Build history of the part. All positions in model axes, mm. A direction names the side the tool comes from. Give positions to 0.01 mm unless a question says otherwise; leave off trailing zeros. Write each loop counter-clockwise with the first axis right and the second up, starting at its lowest first coordinate (ties: lowest second). Pieces come first, ordered by that corner, then holes. Notation, with made-up numbers: M 64.5,52.5 L 90.5,52.5 A21 cw 90.5,57.5 Z; hole C -39,-11.5 d6. An arc over 180 degrees is marked long. Return JSON: item names as keys, results as strings. Group by question number.
Q1. Wall check: probe 1 along X at (y, z) = (36, 8) (3 decimals); probe 2 along Y at (x, z) = (11.1, 0). Give the ranges that are in metal, low to high.
Q2. Band-saw the part on D-D, the plane y = 54. Give the cut face in (x, z) (3 decimals).
Q3. Band-saw the part on C-C, the plane z = 0. Give the cut face in (x, y) (3 decimals), then the cut area to 3 significant figures.
Q4. Band-saw the part on B-B, the plane y = 12.7. Give the cut face in (x, z) (3 decimals), then the cut area to 3 significant figures.
Q5. Pull direction X, two halves, no side cores. Call faces 3 (the flat face through (-12.7, 138, 0)), 4 (the flat face through (0, 138, 9.525)), 5 (the cylindrical face through (-11.09, 15.924, 0.423)): +X half, -X half, draft (parallel to the pull), parting line (faces both ways), or undercut.
Q6. Tool access for faces 1 (the flat face through (12.7, 138, 0)), 2 (the flat face through (0, 138, -9.525)): list every direction of +Z, -Z, +X, -X, +Y, -Y with a clear straight run to the whole face (end or side of a thin tool).
Q7. Flat gauge pins, fed straight in: pin 1 Ø10.5 at (y, z) = (12.7, 0) entering from +X; pin 2 Ø3 at (x, z) = (-6.5, -2.5) entering from -Y (3 decimals). Where does each tip first touch, or does it go through?
Q8. Band-saw the part on A-A, the plane x = -1.75. Give the cut face in (y, z) (3 decimals), then the cut area to 3 significant figures.
Autodesk Inventor part; units mm, degrees
ref_plane "YZ Plane" through (0, 0, 0) normal (1, 0, 0) x (0, 1, 0)
ref_plane "XZ Plane" through (0, 0, 0) normal (0, 1, 0) x (-1, 0, 0)
ref_plane "XY Plane" through (0, 0, 0) normal (0, 0, 1) x (1, 0, 0)
sketch "Sketch1" plane through (0, 0, 0) normal (0, 1, 0) x (-1, 0, 0)
  line L0 (-12.7, -12.7) -> (12.7, -12.7)
  line L1 (12.7, -12.7) -> (12.7, 12.7)
  line L2 (12.7, 12.7) -> (-12.7, 12.7)
  line L3 (-12.7, 12.7) -> (-12.7, -12.7)
  line L4 (-12.7, -12.7) -> (12.7, 12.7) construction
  line L5 (12.7, -12.7) -> (-12.7, 12.7) construction
  line L6 (9.525, 9.525) -> (9.525, -9.525)
  line L7 (9.525, -9.525) -> (-9.525, -9.525)
  line L8 (-9.525, -9.525) -> (-9.525, 9.525)
  line L9 (-9.525, 9.525) -> (9.525, 9.525)
  point P0 (0, 0)
  dimension "d0" = 25.4
  dimension "d1" = 25.4
  dimension "d2" = 3.175
extrude "Extrusion1" add sketch "Sketch1" along normal blind 279.4
sketch "Sketch2" plane through (12.7, 0, 12.7) normal (1, 0, 0) x (0, 0, -1)
  circle A0 centre (12.7, 12.7) radius 3.2512
  line L0 (0, 0) -> (25.4, 0)
  point P0 (12.7, 0)
  point P1 (12.7, 0)
  point P2 (12.7, 0)
  dimension "d5" = 6.5024
  dimension "d6" = 12.7
extrude "Extrusion2" cut sketch "Sketch2" against normal blind 25.4
properties part number "STRU_010_BilletPole_11in_Unique" material "Aluminum 6061"
From the geometry:
{
 "1": {"probe 1": "x = -12.7 to -9.525, 9.525 to 12.7", "probe 2": "y = 0 to 9.45, 15.95 to 279.4"},
 "2": {"outline": "M -12.7,-12.7 L 12.7,-12.7 L 12.7,12.7 L -12.7,12.7 Z; hole M -9.525,-9.525 L 9.525,-9.525 L 9.525,9.525 L -9.525,9.525 Z"},
 "3": {"outline": "M -12.7,0 L -9.525,0 L -9.525,9.449 L -12.7,9.449 Z; M -12.7,15.951 L -9.525,15.951 L -9.525,279.4 L -12.7,279.4 Z; M 9.525,0 L 12.7,0 L 12.7,9.449 L 9.525,9.449 Z; M 9.525,15.951 L 12.7,15.951 L 12.7,279.4 L 9.525,279.4 Z", "area": "1,730 mm^2"},
 "4": {"outline": "M -12.7,-12.7 L 12.7,-12.7 L 12.7,-3.251 L 9.525,-3.251 L 9.525,-9.525 L -9.525,-9.525 L -9.525,-3.251 L -12.7,-3.251 Z; M -12.7,3.251 L -9.525,3.251 L -9.525,9.525 L 9.525,9.525 L 9.525,3.251 L 12.7,3.251 L 12.7,12.7 L -12.7,12.7 Z", "area": "241 mm^2"},
 "5": {"face 3": "-X half", "face 4": "undercut", "face 5": "draft"},
 "6": {"face 1": "+Z, -Z, +X, +Y, -Y", "face 2": "+Y, -Y"},
 "7": {"pin 1": "stops at x = 12.7", "pin 2": "passes through"},
 "8": {"outline": "M 0,-12.7 L 279.4,-12.7 L 279.4,-9.525 L 0,-9.525 Z; M 0,9.525 L 279.4,9.525 L 279.4,12.7 L 0,12.7 Z", "area": "1,770 mm^2"}
}
